Part model, mm, in its own coordinate system. Round coordinates to 2 decimals unless told otherwise and drop trailing zeros. Write each loop counter-clockwise with the first axis right and the second up, starting at its lowest first coordinate (ties: lowest second). Pieces come first, ordered by that corner, then holes. Notation, with made-up numbers: M -13.5,55 L 36.5,55 A35 cw 36.5,90 Z; hole C 24.25,55.5 d10. An arc over 180 degrees is marked long. Use one line per item in the form item = value. Start each with the question number.
Item 1: Probe L1, parallel to X at y = -62, z = 0.4; L2, parallel to X at y = -52, z = 0.5; L3, parallel to Y at x = 7, z = 1. List the from-to ranges inside material, lowest first.
Item 2: Cut at C-C, the plane x = 69. Give the cut face in (y, z), then the cut area to 3 significant figures.
Item 3: Cut at B-B, the plane y = -33.5. Give the cut face in (x, z).
Item 4: Cut at A-A, the plane z = 1.4. Give the cut face in (x, y) (1 decimal).
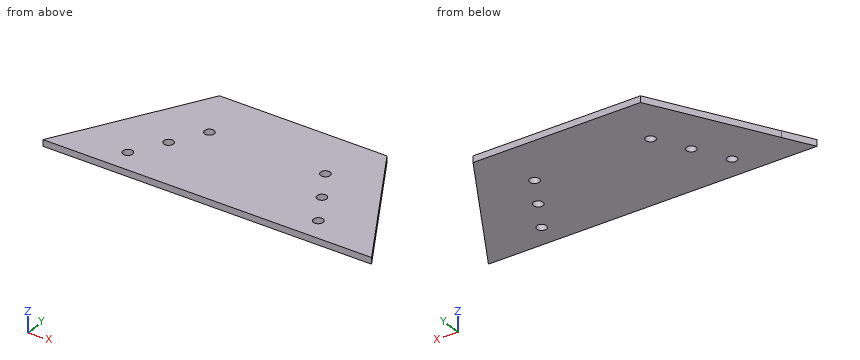
Autodesk Inventor part; units mm, degrees
ref_plane "YZ Plane" through (0, 0, 0) normal (1, 0, 0) x (0, 1, 0)
ref_plane "XZ Plane" through (0, 0, 0) normal (0, 1, 0) x (-1, 0, 0)
ref_plane "XY Plane" through (0, 0, 0) normal (0, 0, 1) x (1, 0, 0)
sketch "スケッチ1" plane through (0, 0, 0) normal (0, 0, 1) x (1, 0, 0)
  line L0 (-21.0154, -61.075) -> (70.9846, -61.075)
  line L1 (70.9846, -61.075) -> (50.9846, -26.434)
  line L2 (50.9846, -26.434) -> (-1.0154, -26.434)
  line L3 (-1.0154, -26.434) -> (-21.0154, -61.075)
  point P0 (0, 0)
  dimension "d0" = 92
  dimension "d1" = 40
  dimension "d2" = 60
  dimension "d3" = 52
extrude "押し出し1" add sketch "スケッチ1" along normal blind 2
sketch "スケッチ2" plane through (0, 0, 2) normal (0, 0, 1) x (1, 0, 0)
  circle A0 centre (6.975, -42.5942) radius 1.5
  line L0 (-1.0154, -26.434) -> (-21.0154, -61.075)
  line L1 (50.9846, -26.434) -> (-1.0154, -26.434)
  line L2 (-1.0154, -26.434) -> (24.9653, -41.434)
  line L3 (-1.0154, -26.434) -> (28.9846, -26.434) construction
  line L4 (70.9846, -61.075) -> (50.9846, -26.434)
  line L5 (50.9846, -26.434) -> (24.9751, -41.4506)
  circle A1 centre (1.2015, -52.5942) radius 1.5
  circle A2 centre (-4.572, -62.5942) radius 1.5
  line L6 (-21.0154, -61.075) -> (70.9846, -61.075)
  line L7 (-21.0154, -61.075) -> (-26.0154, -69.7352)
  line L8 (-21.0154, -61.075) -> (-11.0154, -61.075) construction
  line L9 (-26.0154, -69.7352) -> (75.9846, -69.7352)
  line L10 (75.9846, -69.7352) -> (70.9846, -61.075)
  point P0 (0, 0)
  dimension "d6" = 3
  dimension "d7" = 15
  dimension "d8" = 30
  dimension "d9" = 30
  dimension "d10" = 10
  dimension "d11" = 3
  dimension "d12" = 3
  dimension "d13" = 10
  dimension "d14" = 15
  dimension "d15" = 10
  dimension "d16" = 120
  dimension "d17" = 60
  dimension "d18" = 10
  dimension "d19" = 15
extrude "押し出し2" add sketch "スケッチ2" against normal blind 2 contours L6 L10 L9 L7
sketch "スケッチ3" plane through (0, 0, 2) normal (0, 0, 1) x (1, 0, 0)
  line L0 (-1.0154, -26.434) -> (-26.0154, -69.7352)
  line L1 (-1.0154, -26.434) -> (24.9653, -41.434)
  line L2 (-1.0154, -26.434) -> (28.9846, -26.434) construction
  line L3 (24.9653, -41.434) -> (50.9461, -26.434)
  circle A0 centre (6.975, -42.5942) radius 1.5
  circle A1 centre (1.2015, -52.5942) radius 1.5
  circle A2 centre (42.9846, -42.5776) radius 1.5
  circle A3 centre (48.7581, -52.5776) radius 1.5
  circle A4 centre (54.5316, -62.5776) radius 1.5
  line L4 (75.9846, -69.7352) -> (50.9846, -26.434)
  point P0 (0, 0)
  dimension "d22" = 30
  dimension "d23" = 30
  dimension "d24" = 120
  dimension "d25" = 3
  dimension "d26" = 15
  dimension "d27" = 10
  dimension "d28" = 3
  dimension "d29" = 15
  dimension "d30" = 10
  dimension "d31" = 3
  dimension "d32" = 3
  dimension "d33" = 3
  dimension "d34" = 15
  dimension "d35" = 15
  dimension "d36" = 15
  dimension "d37" = 10
  dimension "d38" = 10
  dimension "d39" = 10
hole "穴1" at (1.2015, -52.5942, 2) at (6.975, -42.5942, 2) at (42.9846, -42.5776, 2) at (54.5316, -62.5776, 2) at (48.7581, -52.5776, 2) direction (0, 0, -1) diameter 3 depth 2
equation "\"BendRadius\" = Thickness"
equation "\"BendReliefWidth\" = Thickness"
equation "\"BendReliefDepth\" = 0.5 * Thickness"
equation "\"CornerReliefSize\" = 4 * Thickness"
equation "\"MinimumRemnant\" = 2 * Thickness"
equation "\"TransitionRadius\" = BendRadius"
equation "\"JacobiRadiusSize\" = BendRadius"
equation "\"GapSize\" = Thickness"
properties part number "nhk22" material "アルミニウム 6061"
Model answer:
q1.L1 = -21.55 to -5.95, -3.19 to 53.15, 55.92 to 71.52
q1.L2 = -15.78 to -0.18, 2.58 to 47.37, 50.14 to 65.75
q1.L3 = -69.74 to -44.09, -41.09 to -26.43
q2.outline = M -69.74,0 L -57.64,0 L -57.64,2 L -69.74,2 Z
q2.area = 24.2 mm²
q3.outline = M -5.09,0 L 55.06,0 L 55.06,2 L -5.09,2 Z
q4.outline = M -26,-69.7 L 76,-69.7 L 71,-61.1 L 51,-26.4 L -1,-26.4 L -21,-61.1 Z; hole C -4.6,-62.6 d3; hole C 1.2,-52.6 d3; hole C 7,-42.6 d3; hole C 43,-42.6 d3; hole C 48.8,-52.6 d3; hole C 54.5,-62.6 d3
